```python
from build123d import *

# Parameters (mm, degrees)
SKETCH1_R           = 5
BOSS_EXTRUDE1_DEPTH = 4
SKETCH2_W           = 4
SKETCH2_H           = 45.7
BOSS_EXTRUDE2_DEPTH = 21.3


with BuildPart() as part:
    # Sketch1 → Boss-Extrude1 (new body)
    with BuildSketch(Plane(origin=(0, 0, 0), x_dir=(1, 0, 0), z_dir=(0, 1, 0))):
        with BuildLine():
            Line((-87.35, -50.5), (87.35, -50.5))
            ThreePointArc((87.35, -50.5), (101.492135624, -44.642135624), (107.35, -30.5))
            Line((107.35, -30.5), (107.35, 30.5))
            ThreePointArc((107.35, 30.5), (101.492135624, 44.642135624), (87.35, 50.5))
            Line((87.35, 50.5), (-87.35, 50.5))
            ThreePointArc((-87.35, 50.5), (-101.492135624, 44.642135624), (-107.35, 30.5))
            Line((-107.35, 30.5), (-107.35, -30.5))
            ThreePointArc((-107.35, -30.5), (-101.492135624, -44.642135624), (-87.35, -50.5))
        make_face()
        with Locations((-92.35, 35.5)):
            Circle(SKETCH1_R, mode=Mode.SUBTRACT)
        with Locations((92.35, 35.5)):
            Circle(SKETCH1_R, mode=Mode.SUBTRACT)
        with Locations((92.35, -35.5)):
            Circle(SKETCH1_R, mode=Mode.SUBTRACT)
        with Locations((-92.35, -35.5)):
            Circle(SKETCH1_R, mode=Mode.SUBTRACT)
    extrude(amount=BOSS_EXTRUDE1_DEPTH)

    # Sketch2 → Boss-Extrude2 (add)
    with BuildSketch(Plane(origin=(0, 4, 0), x_dir=(1, 0, 0), z_dir=(0, 1, 0))):
        with Locations((-105.35, 0)):
            Rectangle(SKETCH2_W, SKETCH2_H)
    extrude(amount=-BOSS_EXTRUDE2_DEPTH)


solid = part.part
```
CAD build for the part. Positions are in the model's coordinates, mm. A direction names the side the tool comes from. Round coordinates to 2 decimals unless told otherwise and drop trailing zeros. Order: outer loops, then holes, each group sorted by start corner. A loop starts at its lowest first (then second) coordinate and runs counter-clockwise, first axis right, second up.
Q1. Which spindle directions (+Z, -Z, +X, -X, +Y, -Y) get a long thin tool onto all of the face, cutting with end or side? Do faces 4 (the flat face through (-103.35, -9, 0)), 5 (the cylindrical face through (101.336, 1.972, 44.797)), 6 (the flat face through (-105, -9, 22.85)), 7 (the flat face through (-105, -9, -22.85)). Say none if no direction does.
Q2. Slice it at D-D (y = -4). Write the cut outline in (x, z).
Q3. Slice it at B-B (z = -0.5). Write the cut outline in (x, y).
Q4. Slice it at C-C (z = -35.5). Write the cut outline in (x, y), and give its area (3 significant figures).
Q5. Drop flat-ended pins along their axis: pin 1 (9 mm diameter, centred on x = -92.35, z = 35.5, fed in from -Y); pin 2 (8.5 mm diameter, centred on y = -11, z = 0, fed in from +X); pin 3 (11.5 mm diameter, centred on x = -92.35, z = -35.5, fed in from -Y); pin 4 (4.5 mm diameter, centred on x = -105.5, y = -5.5, fed in from -Z). Give the stop position or say it passes through.
Q6. Slice it at A-A (x = 92.35). Write the cut outline in (y, z).
Q7. Two-plate mould, pull along X, no slides. Class faces 1 (the cylindrical face through (-97.345, 1.972, -35.72)), 2 (the cylindrical face through (-101.647, 1.972, 44.486)), 3 (the flat face through (-1, 2, 50.5)): pulls with the +X half, pulls with the -X half, needs draft (parallel to the pull), parting line crosses it, or undercut.
Q8. Wall check: L1, parallel to X at y = 2.4, z = -35.5; L2, parallel to Z at x = -90.5, y = 0.25; L3, parallel to Z at x = -92.35, y = 3.25. Give the ranges that are in metal, low to high.
Results below:
1. face 4: +Z, -Z, +X, -Y
1. face 5: +Z, +X, +Y, -Y
1. face 6: +Z, +X, -X, -Y
1. face 7: -Z, +X, -X, -Y
2. outline: (-107.35, -22.85) - (-103.35, -22.85) - (-103.35, 22.85) - (-107.35, 22.85) - close
3. outline: (-107.35, -17.3) - (-103.35, -17.3) - (-103.35, 0) - (107.35, 0) - (107.35, 4) - (-107.35, 4) - close
4. outline: (-106.71, 0) - (-97.35, 0) - (-97.35, 4) - (-106.71, 4) - close; (-87.35, 0) - (87.35, 0) - (87.35, 4) - (-87.35, 4) - close; (97.35, 0) - (106.71, 0) - (106.71, 4) - (97.35, 4) - close
4. area: 774 mm2
5. pin 1: passes through
5. pin 2: stops at x = -103.35
5. pin 3: stops at y = 0
5. pin 4: stops at z = -22.85
6. outline: (0, -49.86) - (4, -49.86) - (4, -40.5) - (0, -40.5) - close; (0, -30.5) - (4, -30.5) - (4, 30.5) - (0, 30.5) - close; (0, 40.5) - (4, 40.5) - (4, 49.86) - (0, 49.86) - close
7. face 1: undercut
7. face 2: pulls with the -X half
7. face 3: needs draft
8. L1: x = -106.71 to -97.35, -87.35 to 87.35, 97.35 to 106.71
8. L2: z = -50.25 to -40.15, -30.85 to 30.85, 40.15 to 50.25
8. L3: z = -49.86 to -40.5, -30.5 to 30.5, 40.5 to 49.86
